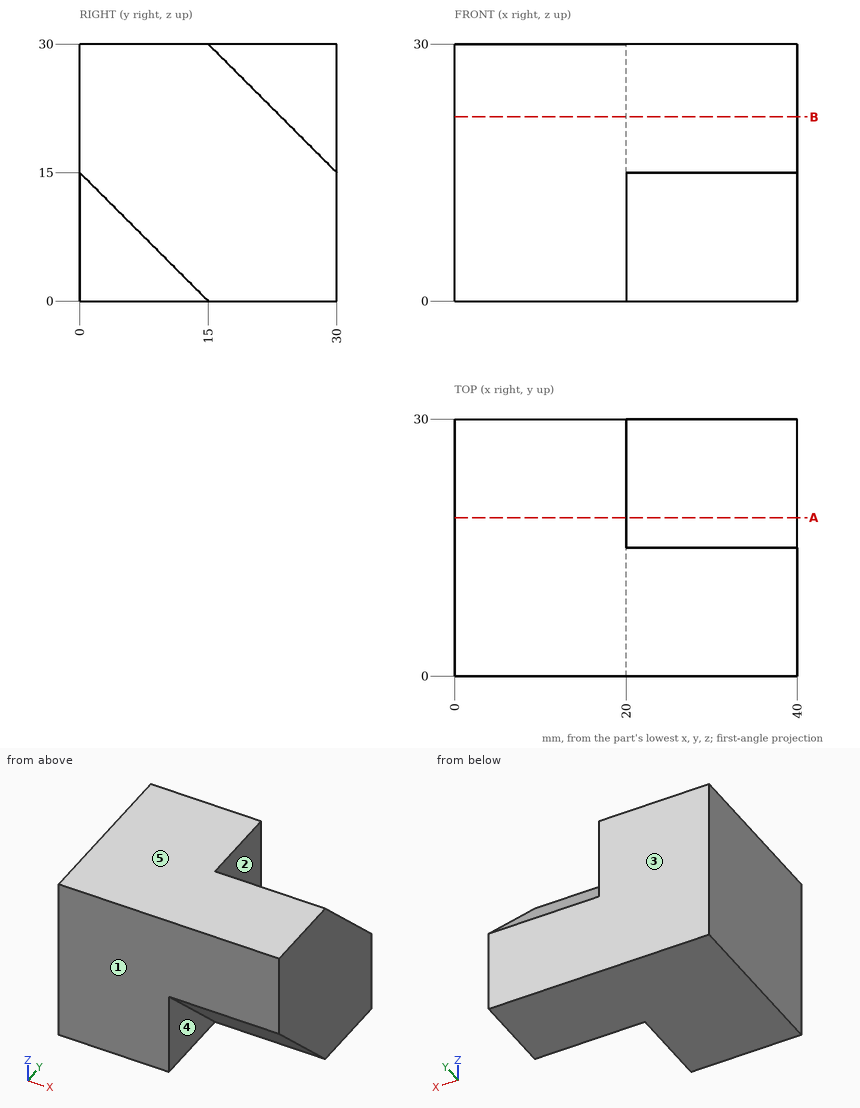
Drawing for the job (mm, zero at the part's lowest x, y, z). A direction names the side the tool comes from. Round coordinates to 2 decimals unless told otherwise and drop trailing zeros. Loops run counter-clockwise (first coordinate to the right, second up) from the corner with the lowest first, then second, coordinate; pieces in that order, holes last. Notation, with made-up numbers: (-5, -20) -> (15, -20) arc R23 cw to (15, 6) -> close; hole circle Ø5 at (76, 16.5). An arc over 180 degrees is marked (long way). Answer in a Markdown table with one row per item.
Item 1: Pin check, flat tip, straight feed: pin 1 (12 mm diameter, centred on x = 31, z = 26, fed in from +Y). Stop position of the tip, or through.
Answers below:
| item | result |
|---|---|
| pin 1 | stops at y = 25 |
Item 2: Mould opens along Y. For the marked faces 1, 2 and 3 say: +Y half, -Y half, draft (parallel to the pull), parting line (faces both ways), or undercut.
Answers below:
| item | result |
|---|---|
| face 1 | -Y half |
| face 2 | draft |
| face 3 | +Y half |
Item 3: Drill centre lines: L1, parallel to X at y = 11, z = 3.5; L2, parallel to Z at x = 31, y = 1.75; L3, parallel to Y at x = 28.5, z = 21. Where is each one in solid material? Low to high. Write a range as [from, to].
Answers below:
| item | result |
|---|---|
| L1 | x = [0, 20] |
| L2 | z = [13.25, 30] |
| L3 | y = [0, 24] |
Item 4: Saw through at A-A (y = 18.5). Write the cut outline in (x, z), and give its area (3 significant figures).
Answers below:
| item | result |
|---|---|
| outline | (0, 0) -> (40, 0) -> (40, 26.5) -> (20, 26.5) -> (20, 30) -> (0, 30) -> close |
| area | 1,130 mm² |
Item 5: Saw through at B-B (z = 21.5). Write the cut outline in (x, y), and give its area (3 significant figures).
Answers below:
| item | result |
|---|---|
| outline | (0, 0) -> (40, 0) -> (40, 23.5) -> (20, 23.5) -> (20, 30) -> (0, 30) -> close |
| area | 1,070 mm² |
Item 6: Which spindle directions (+Z, -Z, +X, -X, +Y, -Y) get a long thin tool onto all of the face, cutting with end or side? Do the marked faces 4 and 5. Say none if no direction does.
Answers below:
| item | result |
|---|---|
| face 4 | -Z, +X, -Y |
| face 5 | +Z, +X, -X, +Y, -Y |
